```python
from build123d import *

# Parameters (mm, degrees)
SKETCH1_W           = 9
SKETCH1_H           = 40
BOSS_EXTRUDE1_DEPTH = 2.5
BOSS_EXTRUDE2_START = -5.25
SKETCH2_R           = 2.5
BOSS_EXTRUDE2_DEPTH = 9.5
SKETCH3_R           = 1.5
CUT_EXTRUDE1_DEPTH  = 42.919565837
SKETCH4_R           = 2.875
CUT_EXTRUDE2_DEPTH  = 5.25
CUT_EXTRUDE3_START  = -14.75
SKETCH4_2_R         = 2.875
CUT_EXTRUDE3_DEPTH  = 5.25
SKETCH5_R           = 1.5
CUT_EXTRUDE4_DEPTH  = 42.695323479
CHAMFER1_SIZE       = 1
CHAMFER2_SIZE       = 1


with BuildPart() as part:
    # Sketch1 → Boss-Extrude1 (new body)
    with BuildSketch(Plane(origin=(0, 0, 0), x_dir=(1, 0, 0), z_dir=(0, 1, 0))):
        with Locations((-4.5, 20)):
            Rectangle(SKETCH1_W, SKETCH1_H)
    extrude(amount=BOSS_EXTRUDE1_DEPTH)

    # Sketch2 → Boss-Extrude2 (add)
    with BuildSketch(Plane.XY.offset(BOSS_EXTRUDE2_START)):
        with Locations((-9, 2.5)):
            Circle(SKETCH2_R)
    boss_extrude2 = extrude(amount=-BOSS_EXTRUDE2_DEPTH)

    # Sketch3 → Cut-Extrude1 (cut, through all)
    with BuildSketch(Plane.XY):
        with Locations((-9, 2.5)):
            Circle(SKETCH3_R)
    cut_extrude1 = extrude(amount=-CUT_EXTRUDE1_DEPTH, mode=Mode.SUBTRACT)

    # Sketch4 → Cut-Extrude2 (cut)
    with BuildSketch(Plane.XY):
        with Locations((-9, 2.5)):
            Circle(SKETCH4_R)
    cut_extrude2 = extrude(amount=-CUT_EXTRUDE2_DEPTH, mode=Mode.SUBTRACT)

    # Sketch4<2> → Cut-Extrude3 (cut)
    with BuildSketch(Plane.XY.offset(CUT_EXTRUDE3_START)):
        with Locations((-9, 2.5)):
            Circle(SKETCH4_2_R)
    cut_extrude3 = extrude(amount=-CUT_EXTRUDE3_DEPTH, mode=Mode.SUBTRACT)

    # Mirror2: Boss-Extrude2, Cut-Extrude1, Cut-Extrude2, Cut-Extrude3 across plane
    add(boss_extrude2.mirror(Plane.XY.offset(-20)))
    add(cut_extrude1.mirror(Plane.XY.offset(-20)), mode=Mode.SUBTRACT)
    add(cut_extrude2.mirror(Plane.XY.offset(-20)), mode=Mode.SUBTRACT)
    add(cut_extrude3.mirror(Plane.XY.offset(-20)), mode=Mode.SUBTRACT)

    # Sketch5 → Cut-Extrude4 (cut, through all)
    with BuildSketch(Plane(origin=(0, 2.5, 0), x_dir=(1, 0, 0), z_dir=(0, 1, 0))):
        with Locations(Location((-3, 10, 0), (0, 0, 270))):
            Circle(SKETCH5_R)
    cut_extrude4 = extrude(amount=-CUT_EXTRUDE4_DEPTH, mode=Mode.SUBTRACT)

    # Mirror3: Cut-Extrude4 across plane
    add(cut_extrude4.mirror(Plane.XY.offset(-20)), mode=Mode.SUBTRACT)

    # Chamfer1
    chamfer1_edges = [part.edges().sort_by_distance(p)[0] for p in [
        (-3, 2.5, -28.5),
    ]]
    chamfer(chamfer1_edges, length=CHAMFER1_SIZE)

    # Chamfer2
    chamfer2_edges = [part.edges().sort_by_distance(p)[0] for p in [
        (-3, 2.5, -11.5),
    ]]
    chamfer(chamfer2_edges, length=CHAMFER2_SIZE)


solid = part.part
```
The listing builds one solid part. Answer for the finished solid, in the listing's coordinates (mm). A direction names the side the tool comes from. Give positions to 0.01 mm unless a question says otherwise; leave off trailing zeros. Order: outer loops, then holes, each group sorted by start corner. A loop starts at its lowest first (then second) coordinate and runs counter-clockwise, first axis right, second up. Notation, with made-up numbers: (73.25, 13) - (88.25, 13) arc R18 cw to (88.25, 29) - close; hole circle Ø1 at (81.5, 67.5). An arc over 180 degrees is marked (long way). Answer in a Markdown table with one row per item. Add a question column.
Q1. The part is cut by section A-A (z = -10). Determine the outline of the cut face in (x, y), then the cut area to 3 significant figures.
Q2. Find the intervals of material crossed by line 1 along Y through (x, z) = (-9, -10); line 2 along X through (y, z) = (1.15, -10); line 3 along Z through (x, y) = (-3.5, 1.6), in increasing order. Write a range as [from, to].
Q3. Given P1, Ø6, axis at x = -5.5, z = -11.5, coming from the +Y side; P2, Ø1.5, axis at x = -8.5, y = 3.5, coming from the -Z side; P3, Ø2.5, axis at x = -3, z = -10, coming from the +Y side; P4, Ø1, axis at y = 1.5, z = -22, coming from the -X side, each flat-ended and moving along its own axis, determine where each tip first touches the part or whether it passes through.
Q4. The part is cut by section D-D (x = -10). Determine the outline of the cut face in (y, z), then the cut area to 3 significant figures.
Q5. For a pull along X with two mould halves and no side action, classify faces 5 (the cylindrical face through (-10.2, 1.6, -9.9)), 6 (the flat face through (-9.45, 0.87, -14.75)), 7 (the cylindrical face through (-6.526, 1.035, -2.588)) as released by +X, released by -X, zero draft, split by the parting line, or undercut.
Q6. Which of the six approach directions +Z, -Z, +X, -X, +Y, -Y give full straight-line access (tool end or side, diameter ignored) to faces 1 (the cylindrical face through (-6.526, 1.035, -37.412)), 2 (the flat face through (-9.45, 0.87, -5.25)), 3 (the flat face through (-9.45, 0.87, -25.25)), 4 (the flat face through (-3, 2.5, -20))?
Q7. The part is cut by section B-B (x = -3). Determine the outline of the cut face in (y, z), then the cut area to 3 significant figures.
Q8. The part is cut by section C-C (y = 3). Determine the outline of the cut face in (x, z), then the cut area to 3 significant figures.
Determined:
| question | item | result |
|---|---|---|
| 1 | outline | (-9, 0) - (-4.5, 0) - (-4.5, 1.5) - (-5.5, 2.5) - (-6.5, 2.5) arc R2.5 ccw (long way) to start; (-1.5, 0) - (0, 0) - (0, 2.5) - (-0.5, 2.5) - (-1.5, 1.5) - close; hole circle Ø3 at (-9, 2.5) |
| 1 | area | 21.7 mm² |
| 2 | line 1 | y = [0, 1], [4, 5] |
| 2 | line 2 | x = [-11.1, -9.65], [-8.35, -4.5], [-1.5, 0] |
| 2 | line 3 | z = [-40, -31.52], [-28.48, -11.52], [-8.48, 0] |
| 3 | P1 | stops at y = 4.95 |
| 3 | P2 | stops at z = -34.75 |
| 3 | P3 | passes through |
| 3 | P4 | stops at x = -6.55 |
| 4 | outline | (0.21, -34.75) - (1.38, -34.75) - (1.38, -25.25) - (0.21, -25.25) - close; (0.21, -14.75) - (1.38, -14.75) - (1.38, -5.25) - (0.21, -5.25) - close; (3.62, -34.75) - (4.79, -34.75) - (4.79, -25.25) - (3.62, -25.25) - close; (3.62, -14.75) - (4.79, -14.75) - (4.79, -5.25) - (3.62, -5.25) - close |
| 4 | area | 44.6 mm² |
| 5 | face 5 | undercut |
| 5 | face 6 | zero draft |
| 5 | face 7 | released by -X |
| 6 | face 1 | -Z, -X, +Y |
| 6 | face 2 | +Z, -X, +Y |
| 6 | face 3 | -X, +Y |
| 6 | face 4 | +Z, -Z, +X, +Y |
| 7 | outline | (0, -40) - (2.5, -40) - (2.5, -32.5) - (1.5, -31.5) - (0, -31.5) - close; (0, -28.5) - (1.5, -28.5) - (2.5, -27.5) - (2.5, -12.5) - (1.5, -11.5) - (0, -11.5) - close; (0, -8.5) - (1.5, -8.5) - (2.5, -7.5) - (2.5, 0) - (0, 0) - close |
| 7 | area | 83.0 mm² |
| 8 | outline | (-11.45, -34.75) - (-10.41, -34.75) - (-10.41, -25.25) - (-11.45, -25.25) - close; (-11.45, -14.75) - (-10.41, -14.75) - (-10.41, -5.25) - (-11.45, -5.25) - close; (-7.59, -34.75) - (-6.55, -34.75) - (-6.55, -25.25) - (-7.59, -25.25) - close; (-7.59, -14.75) - (-6.55, -14.75) - (-6.55, -5.25) - (-7.59, -5.25) - close |
| 8 | area | 39.3 mm² |
